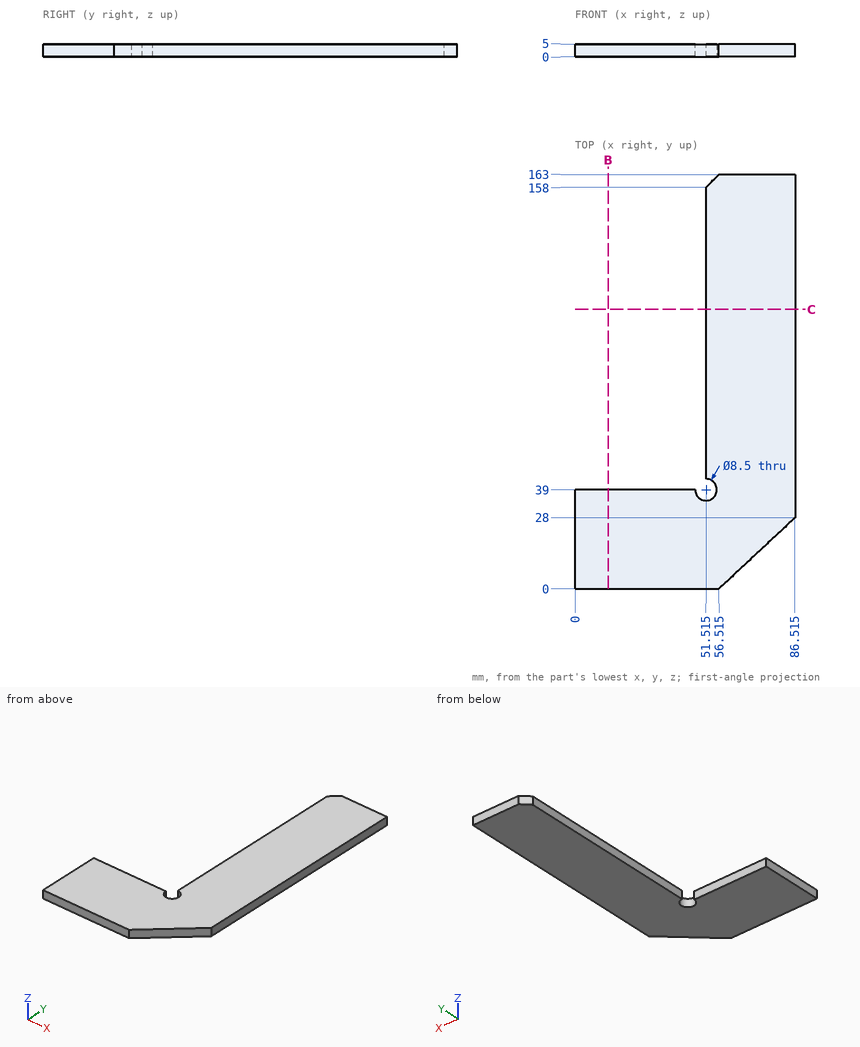
Part print with two shaded views. Sizes in mm from the minimum x, y, z corner. Coordinates: 2 decimals unless noted, no trailing zeros. Order: outer loops, then holes, each group sorted by start corner. A loop starts at its lowest first (then second) coordinate and runs counter-clockwise, first axis right, second up. Notation, with made-up numbers: (-1.5, 81) - (48.5, 81) arc R27 ccw to (48.5, 113) - close; hole circle Ø3 at (-34.5, 31). An arc over 180 degrees is marked (long way). Write item = value, one per line. Start each with the question number.
1) Saw through at B-B on x = 13. Write the cut outline in (y, z), then the cut area to 3 significant figures.
2) Saw through at C-C on y = 110. Write the cut outline in (x, z) (1 decimal).
3) Flat gauge pins, fed straight in: pin 1 Ø1.5 at (y, z) = (81.5, 3) entering from -X (3 decimals); pin 2 Ø2 at (x, z) = (35, 3) entering from +Y; pin 3 Ø7 at (x, y) = (51.52, 39) entering from -Z. Where does each tip first touch, or does it go through?
4) Wall check: line 1 along X through (y, z) = (87.5, 0.2) (1 decimal); line 2 along Y through (x, z) = (29, 1.3); line 3 along Y through (x, z) = (61, 4.2) (1 decimal). Give the ranges that are in metal, low to high. Write a range as from..to.
From the geometry:
q1.outline = (0, 0) - (39, 0) - (39, 5) - (0, 5) - close
q1.area = 195 mm^2
q2.outline = (51.5, 0) - (86.5, 0) - (86.5, 5) - (51.5, 5) - close
q3.pin_1 = 51.515
q3.pin_2 = 39
q3.pin_3 = through
q4.line_1 = 51.5..86.5
q4.line_2 = 0..39
q4.line_3 = 4.2..163
